Solid Edge part; units mm, degrees
sketch "Sketch1" plane through (0, 0, 0) normal (0, 0, 1) x (1, 0, 0)
  line L0 (-7.5, -100) -> (7.5, -100)
  line L1 (7.5, -100) -> (7.5, 100)
  line L2 (7.5, 100) -> (-7.5, 100)
  line L3 (-7.5, 100) -> (-7.5, -100)
  dimension "D1" = 7.5
  dimension "D2" = 7.5
extrude "Protrusion1" add sketch "Sketch1" along normal mid plane 28
hole "Hole_1" at (-7.5, 87.5, 0) direction (1, 0, 0) diameter 14 end up to next counterbore diameter 16 counterbore depth 5 start chamfer 0.6 start chamfer angle 45
hole "Hole1" at (-7.5, -87.5, 0) direction (1, 0, 0) diameter 14 end up to next counterbore diameter 16 counterbore depth 5 start chamfer 0.6 start chamfer angle 45
hole "Hole_3" at (0, 62.5, 14) direction (0, 0, -1) diameter 4.3 depth 30 tip angle 118 start chamfer 0.4 start chamfer angle 45 end chamfer 0.4 end chamfer angle 45
hole "Hole2" at (0, -62.5, 14) direction (0, 0, -1) diameter 4.3 depth 30 tip angle 118 start chamfer 0.4 start chamfer angle 45 end chamfer 0.4 end chamfer angle 45
sketch "Sketch2" plane through (0, 0, 14) normal (0, 0, 1) x (0, -1, 0)
  line L0 (-60, -7.5) -> (-57, -4.5)
  line L1 (-57, -4.5) -> (57, -4.5)
  line L2 (57, -4.5) -> (60, -7.5)
  line L3 (60, -7.5) -> (-60, -7.5)
  dimension "D1" = 60
  dimension "D2" = 57
extrude "Cutout1" cut sketch "Sketch2" against normal up to next
chamfer "Chamfer_1" distance 2.5 angle 45 4 edges at (-7.5, 100, 0) (7.5, 100, 0) (-7.5, -100, 0) (7.5, -100, 0)
sketch "Sketch3" plane through (7.5, 0, 0) normal (1, 0, 0) x (0, 1, 0)
  line L0 (-100, 9) -> (-75, 9)
  line L1 (-75, 9) -> (-70, 14)
  line L2 (-70, 14) -> (-100, 14)
  line L3 (-100, 14) -> (-100, 9)
  dimension "D1" = 70
  dimension "D2" = 100
  dimension "D3" = 100
extrude "Cutout2" cut sketch "Sketch3" against normal up to next
mirror "Mirror1" about plane through (0, 0, 0) normal (0, -1, 0) of "Cutout2"
sketch "Sketch4" plane through (7.5, 0, 0) normal (1, 0, 0) x (0, 1, 0)
  line L0 (-50, 14) -> (-40, -1)
  line L1 (-40, -1) -> (40, -1)
  line L2 (40, -1) -> (50, 14)
  line L3 (50, 14) -> (-50, 14)
  dimension "D1" = 50
  dimension "D2" = 40
  dimension "D3" = 40
extrude "Cutout3" cut sketch "Sketch4" against normal up to next
properties material "Polyethylene, low density"
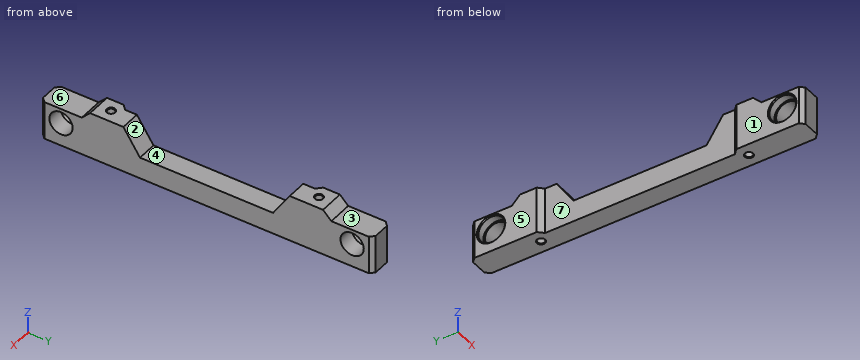
Source: CAD feature listing. Evaluate the final solid. Frame: model axes, mm. Face numbers are marked on the shaded views. A direction names the side the tool comes from. Round coordinates to 2 decimals unless told otherwise and drop trailing zeros. Loops run counter-clockwise (first coordinate to the right, second up) from the corner with the lowest first, then second, coordinate; pieces in that order, holes last. Notation, with made-up numbers: M 50,44 L 85,44 A6 cw 85,55 Z; hole C 39.25,-23 d2. An arc over 180 degrees is marked long. Return JSON: item names as keys, results as strings. Group by question number.
1. Section query B-B on x = 0. State how many separate pieces and enclosed holes the cut face has, and give its area (3 significant figures).
2. Material intervals for line 1 along Y through (x, z) = (3.5, 0.5); line 2 along Z through (x, y) = (-4, -87.5); line 3 along X through (y, z) = (-62.5, 3.25), sorted ascending. Write a range as from..to.
3. Reachability of the marked faces 3, 4, 5, 6 and 7 from +Z, -Z, +X, -X, +Y, -Y: full face, straight path, thin tool, end or side. Return the list, or none.
4. Mould query, pull axis Y, two halves, no side actions, for the marked faces 1 and 2. Classes: released by +Y, released by -Y, zero draft, split by the parting line, or undercut.
5. Pin query (flat end, axial travel): pin 1 (8.5 mm diameter, centred on y = -16, z = -6.5, fed in from -X); pin 2 (1 mm diameter, centred on x = 3, z = 11, fed in from +Y); pin 3 (7.5 mm diameter, centred on x = 2, y = -90, fed in from +Z). Return the tip coordinate at first contact, or that it passes through.
6. Section query A-A on z = 11. Output: boundary loops of the cut face in (x, y), and give its area (3 significant figures).
7. Section query C-C on y = -87.5. Output: boundary loops of the cut face in (x, z).
8. Section query D-D on y = 13. Output: boundary loops of the cut face in (x, z).
Checks:
{
 "1": {"separate pieces": "3", "enclosed holes": "2", "area": "3,430 mm²"},
 "2": {"line 1": "y = -100..-94.48, -80.52..-41, 41..80.52, 94.48..100", "line 2": "z = -14..-8, 8..9", "line 3": "x = -7.5..-2.15, 2.15..7.5"},
 "3": {"face 3": "+Z, +X, -X, +Y", "face 4": "+Z, +X, -X", "face 5": "+Z, -Z, -X, +Y, -Y", "face 6": "+Z, +X, -X, -Y", "face 7": "+Z, -Z, -X"},
 "4": {"face 1": "zero draft", "face 2": "undercut"},
 "5": {"pin 1": "stops at x = -4.5", "pin 2": "stops at y = 73.5", "pin 3": "stops at z = 9"},
 "6": {"outline": "M -7.5,-73 L 7.5,-73 L 7.5,-48 L -4.5,-48 L -4.5,-57 L -7.5,-60 Z; M -7.5,60 L -4.5,57 L -4.5,48 L 7.5,48 L 7.5,73 L -7.5,73 Z; hole C 0,-62.5 d4.3; hole C 0,62.5 d4.3", "area": "658 mm²"},
 "7": {"outline": "M -7.5,-14 L 7.5,-14 L 7.5,-7 L -2.5,-7 L -2.5,-8 L -6.9,-8 L -7.5,-8.6 Z; M -7.5,8.6 L -6.9,8 L -2.5,8 L -2.5,7 L 7.5,7 L 7.5,9 L -7.5,9 Z"},
 "8": {"outline": "M -4.5,-14 L 7.5,-14 L 7.5,-1 L -4.5,-1 Z"}
}
